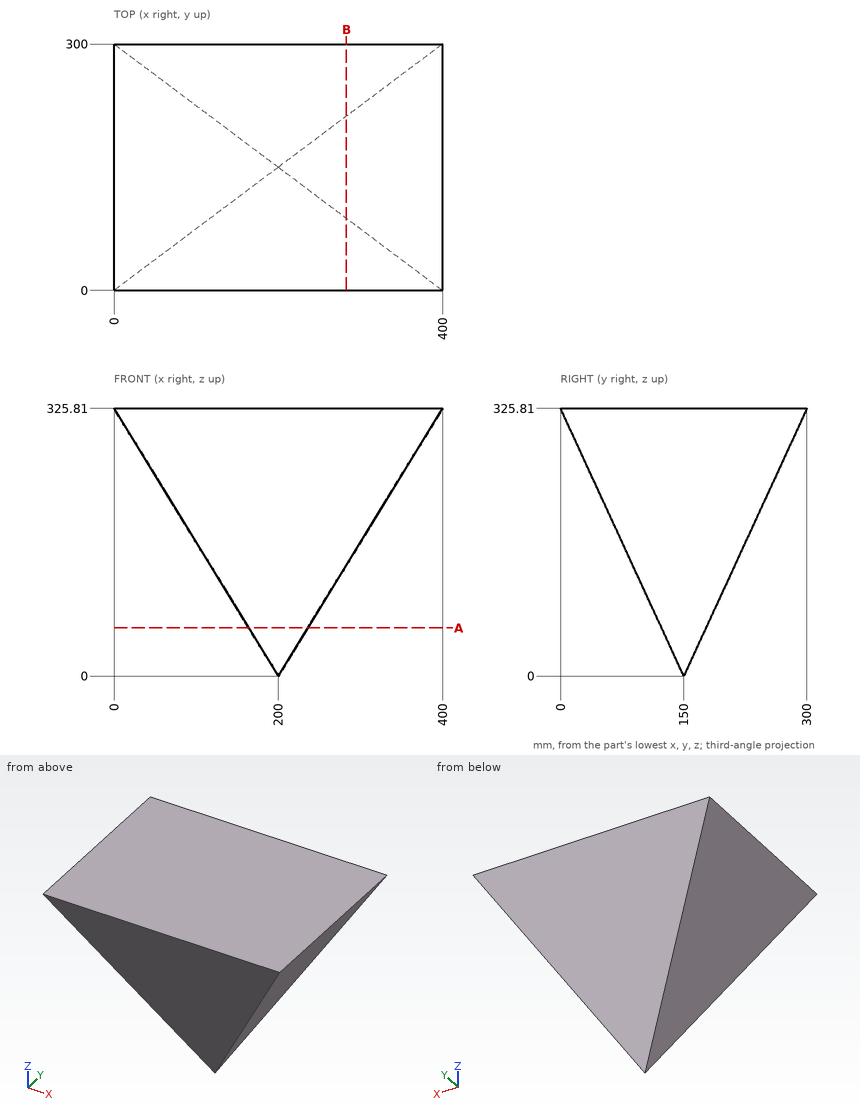
Design review of the part shown in the three views and the two pictorial views. Dimensions are in mm from the part's minimum x, y and z. Round coordinates to 2 decimals unless told otherwise and drop trailing zeros. Write each loop counter-clockwise with the first axis right and the second up, starting at its lowest first coordinate (ties: lowest second). Pieces come first, ordered by that corner, then holes.
1) Take a section at A-A on z = 58.5. Give the boundary of the cut face in (x, y), then the cut area to 3 significant figures.
Answer below:
outline: (164.09, 123.07) - (235.91, 123.07) - (235.91, 176.93) - (164.09, 176.93) - close
area: 3,870 mm2
2) For line 1 along Z through (x, y) = (144.5, 224.5); line 2 along X through (y, z) = (153.5, 270); line 3 along Y through (x, z) = (294.5, 296), list the stretches that pass through material, from the lowest coordinate up.
Answer below:
line 1: z = 161.82 to 325.81
line 2: x = 34.26 to 365.74
line 3: y = 13.72 to 286.28
3) Take a section at B-B on x = 283. Give the boundary of the cut face in (y, z).
Answer below:
outline: (0, 325.81) - (87.75, 135.21) - (212.25, 135.21) - (300, 325.81) - close
4) Insertion check: pin 1 Ø2 at (y, z) = (110, 178) entering from +X; pin 2 Ø10 at (x, z) = (97.5, 240) entering from -Y; pin 3 Ø3 at (x, z) = (332.5, 217.5) entering from -Y. Each pin has a flat end and moves straight along its axis. Give the tip position at first contact, or say it passes through.
Answer below:
pin 1: stops at x = 309.88
pin 2: stops at y = 37.2
pin 3: stops at y = 49.17
